```python
from build123d import *

# Parameters (mm, degrees)
STOCK_NEW_TRACKER_1_START = 60
STOCK_NEW_TRACKER_1_DEPTH = 8
SKETCH1_R                 = 7.509
CUT_EXTRUDE1_DEPTH        = 5
SKETCH2_R                 = 6
CUT_EXTRUDE2_DEPTH        = 143.418251296
BOSS_EXTRUDE1_START       = 1.5
SKETCH6_R                 = 6
BOSS_EXTRUDE1_DEPTH       = 1.5
M4X0_7_TAPPED_HOLE1_D     = 3.3
M4X0_7_TAPPED_HOLE1_DEPTH = 35
M4X0_7_TAPPED_HOLE1_TIP   = 0.991420021


# Read off the part's stored shape, not the designer's step: Stock-New_Tracker-1
with BuildPart() as part:
    # Stock-New_Tracker-1 outline → Stock-New_Tracker-1 (new body)
    with BuildSketch(Plane.YZ.offset(STOCK_NEW_TRACKER_1_START)):
        with BuildLine():
            Line((10, 40), (10, -40))
            Line((10, -40), (96.116983094, -40))
            ThreePointArc((96.116983094, -40), (124.570453884, -28.312888011), (136.594137144, 0))
            ThreePointArc((136.594137144, 0), (124.570453884, 28.312888011), (96.116983094, 40))
            Line((96.116983094, 40), (10, 40))
        make_face()
    extrude(amount=STOCK_NEW_TRACKER_1_DEPTH)

    # Sketch1 → Cut-Extrude1 (cut)
    with BuildSketch(Plane(origin=(68, 0, 0), x_dir=(0, 0, -1), z_dir=(1, 0, 0))):
        with Locations((0, 96.116983094)):
            Circle(SKETCH1_R)
    extrude(amount=-CUT_EXTRUDE1_DEPTH, mode=Mode.SUBTRACT)

    # Sketch2 → Cut-Extrude2 (cut, through all)
    with BuildSketch(Plane(origin=(63, 0, 0), x_dir=(0, 0, -1), z_dir=(1, 0, 0))):
        with Locations((0, 96.116983094)):
            Circle(SKETCH2_R)
    extrude(amount=-CUT_EXTRUDE2_DEPTH, mode=Mode.SUBTRACT)

    # Sketch6 → Boss-Extrude1 (add)
    with BuildSketch(Plane.ZY.offset(-60).offset(BOSS_EXTRUDE1_START)):
        with BuildLine():
            Line((-40, 96.116983094), (-40, 10))
            Line((-40, 10), (40, 10))
            Line((40, 10), (40, 96.116983094))
            ThreePointArc((40, 96.116983094), (28.312888011, 124.570453884), (0, 136.594137144))
            ThreePointArc((0, 136.594137144), (-28.312888011, 124.570453884), (-40, 96.116983094))
        make_face()
        with Locations(Location((0, 96.116983094, 0), (0, 0, 180))):
            Circle(SKETCH6_R, mode=Mode.SUBTRACT)
    extrude(amount=-BOSS_EXTRUDE1_DEPTH)

    # M4x0.7 Tapped Hole1
    with Locations(Plane(origin=(0, 10, 0), x_dir=(-1, 0, 0), z_dir=(0, -1, 0))):
        with Locations((-63.25, -30), (-63.25, 0), (-63.25, 30)):
            Hole(M4X0_7_TAPPED_HOLE1_D / 2, depth=M4X0_7_TAPPED_HOLE1_DEPTH)
            with Locations((0, 0, -(M4X0_7_TAPPED_HOLE1_DEPTH + M4X0_7_TAPPED_HOLE1_TIP / 2))):  # 118° drill point
                Cone(0, M4X0_7_TAPPED_HOLE1_D / 2, M4X0_7_TAPPED_HOLE1_TIP, mode=Mode.SUBTRACT)


solid = part.part
```
Could you check a few things on this model? Use its own coordinates, in mm. A direction names the side the tool comes from. Round coordinates to 2 decimals unless told otherwise and drop trailing zeros. Loops run counter-clockwise (first coordinate to the right, second up) from the corner with the lowest first, then second, coordinate; pieces in that order, holes last. Notation, with made-up numbers: (74.5, 67.5) - (115.5, 67.5) arc R31 ccw to (115.5, 95.5) - close; hole circle Ø4 at (21, 6.25). An arc over 180 degrees is marked (long way). Answer in a Markdown table with one row per item. Add a question column.
(1) If we section it at C-C (z = 14.5): Please give me the cut outline in (x, y), plus the area to 3 significant figures.
(2) If we section it at A-A (y = 22): Please give me the cut outline in (x, z), plus the area to 3 significant figures.
(3) I need wall thicknesses on line 1 along Z through (x, y) = (63.25, 27.5); line 2 along Y through (x, z) = (65.05, 0); line 3 along X through (y, z) = (30, -30). Which ranges of each line are inside material? Lowest first, please.
(4) I'm going to push flat-ended pins straight in: pin 1 (3 mm diameter, centred on x = 63.25, z = 30, fed in from +Y); pin 2 (3 mm diameter, centred on x = 63.25, z = 0, fed in from -Y); pin 3 (1 mm diameter, centred on x = 66.5, z = -6.5, fed in from +Y). Where does each tip first touch, or does it pass through?
(5) For faces 5 (the face through (60.718, 90.168, 0.781)), 6 (the face through (65.54, 103.56, 0.98)), 7 (the face through (62.034, 27.745, -31.115)), which set-ups out of +Z, -Z, +X, -X, +Y, -Y let a thin tool reach every point of the face, with its end or its side?
(6) If we section it at B-B (x = 66.5): Please give me the cut outline in (y, z).
(7) If we mould it in two halves opening along Z, with no side actions, what happens to faces 1 (the face through (63.31, 45.82, -29.72)), 2 (the face through (63, 54, -40)), 3 (the face through (63, 52, 40)), 4 (the face through (68, 72, 1))? For each: pulls with the +Z half, pulls with the -Z half, needs draft (parallel to the pull), parting line crosses it, or undercut.
Model answer:
| question | item | result |
|---|---|---|
| 1 | outline | (58.5, 10) - (68, 10) - (68, 133.72) - (58.5, 133.72) - close |
| 1 | area | 1,180 mm² |
| 2 | outline | (58.5, -40) - (68, -40) - (68, 40) - (58.5, 40) - close; hole circle Ø3.3 at (63.25, -30); hole circle Ø3.3 at (63.25, 0); hole circle Ø3.3 at (63.25, 30) |
| 2 | area | 734 mm² |
| 3 | line 1 | z = -40 to -31.65, -28.35 to -1.65, 1.65 to 28.35, 31.65 to 40 |
| 3 | line 2 | y = 10 to 88.61, 103.63 to 136.59 |
| 3 | line 3 | x = 58.5 to 61.6, 64.9 to 68 |
| 4 | pin 1 | stops at y = 124.38 |
| 4 | pin 2 | stops at y = 45.09 |
| 4 | pin 3 | stops at y = 136.07 |
| 5 | face 5 | +X, -X |
| 5 | face 6 | +X |
| 5 | face 7 | -Y |
| 6 | outline | (10, -40) - (96.12, -40) arc R40.48 ccw to (136.59, 0) arc R40.48 ccw to (96.12, 40) - (10, 40) - close; hole circle Ø15.02 at (96.12, 0) |
| 7 | face 1 | undercut |
| 7 | face 2 | pulls with the -Z half |
| 7 | face 3 | pulls with the +Z half |
| 7 | face 4 | needs draft |
